Check sheet for the modelled part. Datum: model origin and axes. Units: mm. A direction names the side the tool comes from. Coordinates: 2 decimals unless noted, no trailing zeros. Loops run counter-clockwise (first coordinate to the right, second up) from the corner with the lowest first, then second, coordinate; pieces in that order, holes last. Notation, with made-up numbers: (2.25, -32.5) -> (59.25, -32.5) arc R25 ccw to (59.25, -0.5) -> close; hole circle Ø6 at (12, -17). An arc over 180 degrees is marked (long way). Use CSV: the item, a comma, the result in double quotes. Start each with the question number.
1. Sectioned sample at A-A, the plane z = 0. Record the cut outline in (x, y), and give its area (3 significant figures).
2. Release check for a two-part mould opening along Z. For faces 1 (the face through (-1, 3, -77)), 2 (the face through (-8.67, 87.93, -39.05)), 3 (the face through (-1, 39, 60)), 4 (the face through (-1, 44, 63)) record: pulls with the +Z half, pulls with the -Z half, needs draft (parallel to the pull), parting line crosses it, or undercut.
3. Sectioned sample at D-D, the plane x = 0. Record the cut outline in (y, z).
4. Thickness scan on L1, parallel to Z at x = -35, y = 1.05; L2, parallel to X at y = 0.75, z = -80; L3, parallel to Z at x = 0, y = 81.05. Record the ranges inside material, lowest first.
5. Set-up check for faces 5 (the face through (-15, 83, 14)), 6 (the face through (-1, 42, -63)), 7 (the face through (-1, 3, 76)): record each of +Z, -Z, +X, -X, +Y, -Y from which the full face is reachable in a straight line by a thin tool's end or side.
6. Gauge pin test, flat ends, axial feed: pin 1 (9 mm diameter, centred on x = 35, z = -80, fed in from +Y); pin 2 (3 mm diameter, centred on x = -9.5, y = 49, fed in from -Z); pin 3 (13.5 mm diameter, centred on x = -24, z = 70.5, fed in from +Y); pin 4 (5 mm diameter, centred on x = -16, z = -50, fed in from +Y). Record the tip position at first contact, or that the pin passes through.
7. Sectioned sample at B-B, the plane z = -80. Record the cut outline in (x, y).
8. Sectioned sample at C-C, the plane y = 61. Record the cut outline in (x, z).
Autodesk Inventor part; units mm, degrees
ref_plane "YZ Plane" through (0, 0, 0) normal (1, 0, 0) x (0, 1, 0)
ref_plane "XZ Plane" through (0, 0, 0) normal (0, 1, 0) x (-1, 0, 0)
ref_plane "XY Plane" through (0, 0, 0) normal (0, 0, 1) x (1, 0, 0)
sketch "Schizzo1" plane through (0, 0, 0) normal (1, 0, 0) x (0, 1, 0)
  line L0 (0, 90) -> (0, 60)
  line L1 (0, 60) -> (80, 60)
  line L2 (80, 60) -> (80, -60)
  line L3 (80, -60) -> (0, -60)
  line L4 (0, -60) -> (0, -90)
  line L5 (0, -90) -> (3, -90)
  line L6 (3, -90) -> (3, -63)
  line L7 (3, -63) -> (83, -63)
  line L8 (83, -63) -> (83, 63)
  line L9 (83, 63) -> (3, 63)
  line L10 (3, 63) -> (3, 90)
  line L11 (3, 90) -> (0, 90)
  line L12 (0, 0) -> (59.7399, 0) construction
  line L13 (0, 0) -> (0, -69.3642) construction
  dimension "d0" = 30
  dimension "d1" = 120
  dimension "d2" = 3
  dimension "d3" = 3
  dimension "d4" = 83
  dimension "d5" = 3
extrude "Estrusione1" add sketch "Schizzo1" along normal mid plane 100
sketch "Schizzo2" plane through (-50, 83, 63) normal (0, 1, 0) x (1, 0, 0)
  circle A0 centre (50, 63) radius 40
  circle A1 centre (50, 63) radius 32.5
  circle A2 centre (50, 63) radius 20
  dimension "d8" = 80
  dimension "d9" = 65
  dimension "d10" = 40
extrude "Estrusione2" cut sketch "Schizzo2" against normal through all contours A2
extrude "Estrusione3" add sketch "Schizzo2" along normal blind 10 contours A0
sketch "Schizzo3" plane through (-50, 3, 90) normal (0, 1, 0) x (1, 0, 0)
  line L0 (100, 0) -> (100, 30)
  line L1 (100, 30) -> (0, 30)
  line L2 (0, 150) -> (100, 150)
  line L3 (100, 150) -> (100, 180)
  line L4 (0, 180) -> (100, 180)
  line L5 (0, 0) -> (100, 0)
  line L6 (0, 30) -> (0, 0)
  line L7 (0, 180) -> (0, 150)
  line L8 (100, 0) -> (85, 0)
  line L9 (85, 0) -> (85, 10)
  circle A0 centre (85, 10) radius 5
  circle A1 centre (85, 170) radius 5
  circle A2 centre (15, 10) radius 5
  circle A3 centre (15, 170) radius 5
  point P0 (50, 90)
  dimension "d15" = 15
  dimension "d16" = 10
  dimension "d17" = 10
  dimension "d20" = 160
  dimension "d23" = 70
extrude "Estrusione4" cut sketch "Schizzo3" against normal through all contours A0 | A1 | A2 | A3
sketch "Schizzo4" plane through (-50, 3, 90) normal (0, 1, 0) x (1, 0, 0)
  point P0 (50, 90)
sketch "Schizzo5" plane through (-50, 3, 90) normal (0, 1, 0) x (1, 0, 0)
  point P0 (50, 90)
properties part number "Sanson_Amedeo Analisi FEM 2"
Completed:
1,outline,"(-50, 80) -> (-20, 80) -> (-20, 83) -> (-32.5, 83) -> (-32.5, 93) -> (-40, 93) -> (-40, 83) -> (-50, 83) -> close; (20, 80) -> (50, 80) -> (50, 83) -> (40, 83) -> (40, 93) -> (32.5, 93) -> (32.5, 83) -> (20, 83) -> close"
1,area,"330 mm²"
2,face 1,"needs draft"
2,face 2,"parting line crosses it"
2,face 3,"undercut"
2,face 4,"pulls with the +Z half"
3,outline,"(0, -90) -> (3, -90) -> (3, -63) -> (83, -63) -> (83, -40) -> (93, -40) -> (93, -32.5) -> (83, -32.5) -> (83, -20) -> (80, -20) -> (80, -60) -> (0, -60) -> close; (0, 60) -> (80, 60) -> (80, 20) -> (83, 20) -> (83, 32.5) -> (93, 32.5) -> (93, 40) -> (83, 40) -> (83, 63) -> (3, 63) -> (3, 90) -> (0, 90) -> close"
4,L1,"-90 to -85, -75 to -60, 60 to 75, 85 to 90"
4,L2,"-50 to -40, -30 to 30, 40 to 50"
4,L3,"-63 to -20, 20 to 63"
5,face 5,"+Y"
5,face 6,"-Z, +X, -X, +Y"
5,face 7,"+Z, +X, -X, +Y"
6,pin 1,"through"
6,pin 2,"z = -63"
6,pin 3,"y = 3"
6,pin 4,"y = 83"
7,outline,"(-50, 0) -> (-40, 0) -> (-40, 3) -> (-50, 3) -> close; (-30, 0) -> (30, 0) -> (30, 3) -> (-30, 3) -> close; (40, 0) -> (50, 0) -> (50, 3) -> (40, 3) -> close"
8,outline,"(-50, -63) -> (50, -63) -> (50, -60) -> (-50, -60) -> close; (-50, 60) -> (50, 60) -> (50, 63) -> (-50, 63) -> close"
